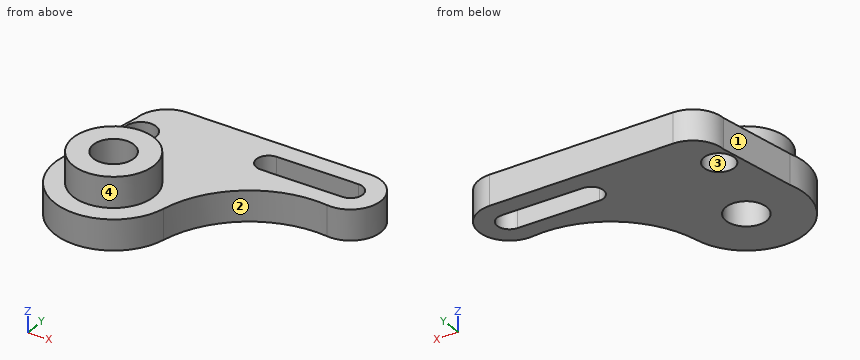
```python
from build123d import *

# Parameters (mm, degrees)
BOSS_EXTRUDE2_DEPTH = 15
SKETCH2_R           = 20
BOSS_EXTRUDE3_DEPTH = 35
SKETCH3_R           = 10
CUT_EXTRUDE2_DEPTH  = 51
SKETCH6_R           = 20
CUT_EXTRUDE3_DEPTH  = 20
SKETCH7_R           = 7.5
CUT_EXTRUDE4_DEPTH  = 31


with BuildPart() as part:
    # Sketch1 → Boss-Extrude2 (new body)
    with BuildSketch(Plane.XY):
        with BuildLine():
            Line((84.958136085, 62.963493234), (-5.041863915, 62.963493234))
            ThreePointArc((-5.041863915, 62.963493234), (-15.648465633, 58.570094952), (-20.041863915, 47.963493234))
            Line((-20.041863915, 47.963493234), (-27.527219981, 9.333410593))
            ThreePointArc((-27.527219981, 9.333410593), (-7.728043394, -28.020309393), (28.419860478, -6.096878185))
            ThreePointArc((28.419860478, -6.096878185), (48.225361717, 24.087490733), (83.192615122, 33.067757746))
            ThreePointArc((83.192615122, 33.067757746), (99.932047269, 47.079194733), (84.958136085, 62.963493234))
        make_face()
        with BuildLine():
            ThreePointArc((45, 41.684539724), (38.958282136, 47.642529759), (44.91627217, 53.684247623))
            Line((44.91627217, 53.684247623), (84.91627217, 53.963347184))
            ThreePointArc((84.91627217, 53.963347184), (90.957990034, 48.005357149), (85, 41.963639285))
            Line((85, 41.963639285), (45, 41.684539724))
        make_face(mode=Mode.SUBTRACT)
    extrude(amount=BOSS_EXTRUDE2_DEPTH)

    # Sketch2 → Boss-Extrude3 (add)
    with BuildSketch(Plane.XY.offset(15)):
        Circle(SKETCH2_R)
    extrude(amount=BOSS_EXTRUDE3_DEPTH)

    # Sketch3 → Cut-Extrude2 (cut, through all)
    with BuildSketch(Plane.XY.offset(50)):
        Circle(SKETCH3_R)
    extrude(amount=-CUT_EXTRUDE2_DEPTH, mode=Mode.SUBTRACT)

    # Sketch6 → Cut-Extrude3 (cut)
    with BuildSketch(Plane.XY.offset(50)):
        Circle(SKETCH6_R)
    extrude(amount=-CUT_EXTRUDE3_DEPTH, mode=Mode.SUBTRACT)

    # Sketch7 → Cut-Extrude4 (cut, through all)
    with BuildSketch(Plane.XY.offset(30)):
        with Locations((-12.716641072, 40)):
            Circle(SKETCH7_R)
    extrude(amount=-CUT_EXTRUDE4_DEPTH, mode=Mode.SUBTRACT)


solid = part.part
```
Verification items for the finished model (mm, model axes). Face numbers are marked on the shaded views. Round coordinates to 2 decimals unless told otherwise and drop trailing zeros. Write each loop counter-clockwise with the first axis right and the second up, starting at its lowest first coordinate (ties: lowest second). Pieces come first, ordered by that corner, then holes. Notation, with made-up numbers: (-28.5, -11.5) -> (13.5, -11.5) arc R24 cw to (13.5, 4.5) -> close; hole circle Ø11 at (-29, -24). An arc over 180 degrees is marked (long way). Write each question's results on one line, items separated by ' | '.
Q1. Draft check along Y on the marked faces 1, 2, 3 and 4. Enter one of: released by +Y, released by -Y, zero draft, split by the parting line, or undercut.
Derived:
face 1: released by +Y | face 2: released by -Y | face 3: undercut | face 4: split by the parting line
Q2. Go/stop test with flat-tipped pins: pin 1 Ø8 at (y, z) = (42, 17.5) entering from +X; pin 2 Ø16 at (x, y) = (0, 0) entering from -Z; pin 3 Ø12 at (x, z) = (21.5, 20.5) entering from -Y; pin 4 Ø10 at (x, y) = (32, 19) entering from +Z. Record where each tip stops, or that it passes through.
Derived:
pin 1: stops at x = 99.69 | pin 2: passes through | pin 3: stops at y = -21.91 | pin 4: stops at z = 15
Q3. Thickness scan on probe 1 along Y at (x, z) = (0, 17); probe 2 along Y at (x, z) = (0, 13.5); probe 3 along X at (y, z) = (1.5, 15.5). Record the ranges inside material, lowest first.
Derived:
probe 1: y = -20 to -10, 10 to 20 | probe 2: y = -29.07 to -10, 10 to 62.96 | probe 3: x = -19.94 to -9.89, 9.89 to 19.94
Q4. Sectioned sample at A-A, the plane x = 6. Record the boundary of the cut face in (y, z).
Derived:
outline: (-28.44, 0) -> (-8, 0) -> (-8, 30) -> (-19.08, 30) -> (-19.08, 15) -> (-28.44, 15) -> close; (8, 0) -> (62.96, 0) -> (62.96, 15) -> (19.08, 15) -> (19.08, 30) -> (8, 30) -> close
Q5. Sectioned sample at C-C, the plane z = 26.25. Record the boundary of the cut face in (x, y), and give its area (3 significant figures).
Derived:
outline: circle Ø40 at (0, 0); hole circle Ø20 at (0, 0) | area: 942 mm²
Q6. Sectioned sample at D-D, the plane z = 11.75. Record the boundary of the cut face in (x, y).
Derived:
outline: (-27.53, 9.33) arc R29.07 ccw (long way) to (28.42, -6.1) arc R50 cw to (83.19, 33.07) arc R15 ccw (long way) to (84.96, 62.96) -> (-5.04, 62.96) arc R15 ccw to (-20.04, 47.96) -> close; hole circle Ø15 at (-12.72, 40); hole circle Ø20 at (0, 0); hole (44.92, 53.68) arc R6 ccw to (45, 41.68) -> (85, 41.96) arc R6 ccw to (84.92, 53.96) -> close
Q7. Sectioned sample at B-B, the plane y = 50.5. Record the boundary of the cut face in (x, z), and give its area (3 significant figures).
Derived:
outline: (-19.83, 0) -> (39.66, 0) -> (39.66, 15) -> (-19.83, 15) -> close; (90.4, 0) -> (99.74, 0) -> (99.74, 15) -> (90.4, 15) -> close | area: 1,030 mm²
